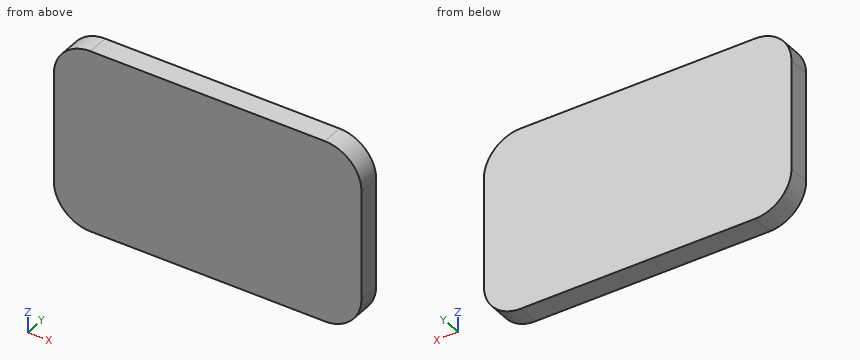
Autodesk Inventor part; units mm, degrees
ref_plane "YZ Plane" through (0, 0, 0) normal (1, 0, 0) x (0, 1, 0)
ref_plane "XZ Plane" through (0, 0, 0) normal (0, 1, 0) x (-1, 0, 0)
ref_plane "XY Plane" through (0, 0, 0) normal (0, 0, 1) x (1, 0, 0)
sketch "Sketch1" plane through (0, 0, 0) normal (0, 1, 0) x (-1, 0, 0)
  line L0 (0, -5) -> (32, -5)
  line L1 (37, 0) -> (37, 15)
  line L2 (32, 20) -> (0, 20)
  line L3 (-5, 15) -> (-5, 0)
  arc A0 (0, 20) -> (-5, 15) centre (0, 15) ccw
  arc A1 (37, 15) -> (32, 20) centre (32, 15) ccw
  arc A2 (32, -5) -> (37, 0) centre (32, 0) ccw
  arc A3 (-5, 0) -> (0, -5) centre (0, 0) ccw
  point P0 (0, 0)
  point P1 (-5, -5)
  point P2 (37, -5)
  point P3 (-5, 20)
  dimension "d0" = 5
  dimension "d1" = 42
  dimension "d2" = 25
  dimension "d3" = 5
  dimension "d4" = 5
extrude "Extrusion1" add sketch "Sketch1" along normal blind 3
properties part number "Bottom Block"
Read the model definition and answer for the solid it produces. Units are mm, in the model's axes. Round coordinates to 2 decimals unless told otherwise and drop trailing zeros. Loops run counter-clockwise (first coordinate to the right, second up) from the corner with the lowest first, then second, coordinate; pieces in that order, holes last.
Q1. Section B-B on z = 17 is taken. Write down the section's boundary in (x, y), and give its area (3 significant figures).
Q2. Section A-A on y = 1.7 is taken. Write down the section's boundary in (x, z), and give its area (3 significant figures).
Q3. This flat-tipped pin is pushed along its axis until it touches: pin 1 (1.5 mm diameter, centred on y = 2, z = 16.5, fed in from +X). Where does it stop, or does it pass through?
Q4. Consider probe 1 along X at (y, z) = (0.8, 17.5); probe 2 along X at (y, z) = (2.55, 15.5); probe 3 along Z at (x, y) = (-33.5, 2.5). Determine where each line is inside the solid, lowest interval first.
Output:
1. outline: (-36.58, 0) - (4.58, 0) - (4.58, 3) - (-36.58, 3) - close
1. area: 123 mm2
2. outline: (-37, 0) arc R5 ccw to (-32, -5) - (0, -5) arc R5 ccw to (5, 0) - (5, 15) arc R5 ccw to (0, 20) - (-32, 20) arc R5 ccw to (-37, 15) - close
2. area: 1,030 mm2
3. pin 1: stops at x = 4.94
4. probe 1: x = -36.33 to 4.33
4. probe 2: x = -36.97 to 4.97
4. probe 3: z = -4.77 to 19.77
